Autodesk Inventor part; units mm, degrees
ref_plane "YZ Plane" through (0, 0, 0) normal (1, 0, 0) x (0, 1, 0)
ref_plane "XZ Plane" through (0, 0, 0) normal (0, 1, 0) x (-1, 0, 0)
ref_plane "XY Plane" through (0, 0, 0) normal (0, 0, 1) x (1, 0, 0)
sketch "Skizze1" plane through (0, 0, 0) normal (1, 0, 0) x (0, 1, 0)
  line L0 (14, 14) -> (-14, 14)
  line L1 (-14, 14) -> (-14, -14)
  line L2 (-14, -14) -> (14, -14)
  line L3 (14, -14) -> (14, 14)
  line L4 (14, 14) -> (-14, -14) construction
  line L5 (-14, 14) -> (14, -14) construction
  line L6 (17, 17) -> (-17, 17)
  line L7 (-17, 17) -> (-17, -17)
  line L8 (-17, -17) -> (17, -17)
  line L9 (17, -17) -> (17, 17)
  line L10 (17, 17) -> (-17, -17) construction
  line L11 (-17, 17) -> (17, -17) construction
  line L12 (-25, 30) -> (30, 30)
  line L13 (30, 30) -> (30, -30)
  line L14 (30, -30) -> (-25, -30)
  line L15 (-25, -30) -> (-25, 30)
  point P0 (0, 0)
  dimension "d0" = 28
  dimension "d1" = 28
  dimension "d2" = 34
  dimension "d3" = 34
  dimension "d4" = 55
  dimension "d5" = 60
extrude "Extrusion1" add sketch "Skizze1" along normal blind 13 contours L3 L2 L1 L0 | L9 L8 L7 L6
sketch "Skizze2" plane through (13, 0, 0) normal (1, 0, 0) x (0, 0, -1)
  point P0 (0, 0)
extrude "Extrusion2" add sketch "Skizze1" along normal blind 5 contours L12 L13 L14 L15
hole "Bohrung1" at (0, 14, -14) at (0, -14, 14) at (0, -14, -14) direction (1, 0, 0) diameter 14 end through all
properties part number "Cube_Insert_Motion_adapter_srew"
Geometry check sheet. Reference: the model listing, model coordinates, mm. A direction names the side the tool comes from. Coordinates: 2 decimals unless noted, no trailing zeros. Loops run counter-clockwise (first coordinate to the right, second up) from the corner with the lowest first, then second, coordinate; pieces in that order, holes last. Notation, with made-up numbers: (10, 83.5) - (20, 83.5) arc R36 cw to (20, 119.5) - close; hole circle Ø2 at (-32, 32.5). An arc over 180 degrees is marked (long way). One line per item, written item: value. Start each with the question number.
(1) Cross-section at B-B on y = -14. Enter the section's corners in (x, z), plus the area to 3 significant figures.
(2) Depth check by flat-ended pin: P1, Ø6, axis at y = 23.5, z = -4, coming from the +X side; P2, Ø3, axis at x = 9, z = 2.5, coming from the -Y side; P3, Ø4, axis at x = 11, y = 3, coming from the +Z side. Enter the tip coordinate at first touch or a pass-through.
(3) Cross-section at A-A on y = 14. Enter the section's corners in (x, z).
(4) Cross-section at D-D on x = 2.75. Enter the section's corners in (y, z), plus the area to 3 significant figures.
(5) Mould release check, pull along Y, two halves, no side actions. Record for faces 6 (the cylindrical face through (5.147, 11.897, -7.323)), 7 (the flat face through (13, 0, 0)), 8 (the flat face through (9, 17, 4)): released by +Y, released by -Y, zero draft, split by the parting line, or undercut.
(6) Tool access check on faces 1 (the flat face through (9, -17, 0)), 2 (the flat face through (2, -25, 0)), 3 (the flat face through (9, 5, 17)), 4 (the flat face through (9, 0, -17)), 5 (the flat face through (0, 2, 0)). Record the directions out of +Z, -Z, +X, -X, +Y, -Y that give a thin tool (end or side, any length) a straight path to the whole face; none if there is none.
(7) Cross-section at C-C on z = 14. Enter the section's corners in (x, y).
(8) Material ranges on line 1 (Z direction, x = 4.5, y = -14); line 2 (Y direction, x = 2.75, z = -14); line 3 (Z direction, x = 9.5, y = -14), recorded low to high. Write a range as [from, to].
Results below:
1. outline: (0, -30) - (5, -30) - (5, -21) - (0, -21) - close; (0, -7) - (13, -7) - (13, 7) - (0, 7) - close; (0, 21) - (5, 21) - (5, 30) - (0, 30) - close
1. area: 272 mm2
2. P1: stops at x = 5
2. P2: stops at y = -17
2. P3: stops at z = 17
3. outline: (0, -30) - (5, -30) - (5, -21) - (0, -21) - close; (0, -7) - (13, -7) - (13, 17) - (5, 17) - (5, 30) - (0, 30) - close
4. outline: (-25, -30) - (30, -30) - (30, 30) - (-25, 30) - close; hole circle Ø14 at (-14, -14); hole circle Ø14 at (-14, 14); hole circle Ø14 at (14, -14)
4. area: 2,840 mm2
5. face 6: undercut
5. face 7: zero draft
5. face 8: released by +Y
6. face 1: +Z, -Z, +X, -Y
6. face 2: +Z, -Z, +X, -X, -Y
6. face 3: +Z, +X, +Y, -Y
6. face 4: -Z, +X, +Y, -Y
6. face 5: +Z, -Z, -X, +Y, -Y
7. outline: (0, -25) - (5, -25) - (5, -21) - (0, -21) - close; (0, -7) - (13, -7) - (13, 17) - (5, 17) - (5, 30) - (0, 30) - close
8. line 1: z = [-30, -21], [-7, 7], [21, 30]
8. line 2: y = [-25, -21], [-7, 7], [21, 30]
8. line 3: z = [-7, 7]
